Source: CAD feature listing. Evaluate the final solid. Frame: model axes, mm. A direction names the side the tool comes from. Coordinates: 2 decimals unless noted, no trailing zeros. Order: outer loops, then holes, each group sorted by start corner. A loop starts at its lowest first (then second) coordinate and runs counter-clockwise, first axis right, second up.
```python
from build123d import *

# Parameters (mm, degrees)
F1_DEPTH = 25.4
F3_DEPTH = 12.701
F5_DEPTH = 12.701


with BuildPart() as f1:
    # F0 (on Front) → F1 (new body)
    with BuildSketch(Plane.XZ):
        Polygon((-34.6547834919, 44.45), (-34.6547834919, 0), (22.4952165081, 0), (22.4952165081, 12.7), (-21.9547834919, 12.7), (-21.9547834919, 44.45), align=None)
    extrude(amount=F1_DEPTH)

    # F2 (on face) → F3 (cut, through all)
    with BuildSketch(Plane.XY.offset(12.7)):
        with BuildLine():
            ThreePointArc((-2.9047834919, -12.7), (-4.7646554313, -8.2098719395), (-9.2547834919, -6.35))
            Line((-9.2547834919, -6.35), (-9.2547834919, -19.05))
            ThreePointArc((-9.2547834919, -19.05), (-4.7646554313, -17.1901280605), (-2.9047834919, -12.7))
        make_face()
        with BuildLine():
            Line((-9.2547834919, -19.05), (-9.2547834919, -6.35))
            ThreePointArc((-9.2547834919, -6.35), (-15.6047834919, -12.7), (-9.2547834919, -19.05))
        make_face()
        with BuildLine():
            Line((9.7952165081, -19.05), (9.7952165081, -6.35))
            ThreePointArc((9.7952165081, -6.35), (3.4452165081, -12.7), (9.7952165081, -19.05))
        make_face()
        with BuildLine():
            ThreePointArc((16.1452165081, -12.7), (14.2853445687, -8.2098719395), (9.7952165081, -6.35))
            Line((9.7952165081, -6.35), (9.7952165081, -19.05))
            ThreePointArc((9.7952165081, -19.05), (14.2853445687, -17.1901280605), (16.1452165081, -12.7))
        make_face()
        with BuildLine():
            Line((22.4952165081, 0), (9.7952165081, 0))
            ThreePointArc((9.7952165081, 0), (18.7754726014, -3.7197438511), (22.4952165081, -12.6999999213))
            Line((22.4952165081, -12.6999999213), (22.4952165081, 0))
        make_face()
        with BuildLine():
            Line((22.4952165081, -25.4), (22.4952165081, -12.6999999213))
            ThreePointArc((22.4952165081, -12.6999999213), (18.775472657, -21.6802560932), (9.7952165081, -25.4))
            Line((9.7952165081, -25.4), (22.4952165081, -25.4))
        make_face()
    extrude(amount=-F3_DEPTH, mode=Mode.SUBTRACT)

    # F4 (on face) → F5 (cut, through all)
    with BuildSketch(Plane.YZ.offset(-21.9547834919)):
        with BuildLine():
            Line((-19.05, 42.7485226281), (-19.05, 31.75))
            ThreePointArc((-19.05, 31.75), (-12.7, 38.1), (-6.35, 31.75))
            Line((-6.35, 31.75), (-6.35, 42.7485226281))
            ThreePointArc((-6.35, 42.7485226281), (-9.4129981272, 44.0172579939), (-12.7, 44.45))
            ThreePointArc((-12.7, 44.45), (-15.9870018728, 44.0172579939), (-19.05, 42.7485226281))
        make_face()
        with BuildLine():
            Line((-25.4, 44.45), (-25.4, 31.75))
            ThreePointArc((-25.4, 31.75), (-23.6985226281, 38.1), (-19.05, 42.7485226281))
            ThreePointArc((-19.05, 42.7485226281), (-15.9870018728, 44.0172579939), (-12.7, 44.45))
            Line((-12.7, 44.45), (-25.4, 44.45))
        make_face()
        with BuildLine():
            Line((0, 44.45), (-12.7, 44.45))
            ThreePointArc((-12.7, 44.45), (-9.4129981272, 44.0172579939), (-6.35, 42.7485226281))
            ThreePointArc((-6.35, 42.7485226281), (-1.7014773719, 38.1), (0, 31.75))
            Line((0, 31.75), (0, 44.45))
        make_face()
        with BuildLine():
            ThreePointArc((-6.35, 31.75), (-12.7, 38.1), (-19.05, 31.75))
            Line((-19.05, 31.75), (-6.35, 31.75))
        make_face()
        with BuildLine():
            Line((-6.35, 31.75), (-19.05, 31.75))
            ThreePointArc((-19.05, 31.75), (-12.7, 25.4), (-6.35, 31.75))
        make_face()
    extrude(amount=-F5_DEPTH, mode=Mode.SUBTRACT)


solid = f1.part
```
1. Draft query along Y for faces 3 (the cylindrical face through (-28.22, -1.75, 38.18)), 4 (the flat face through (-28, -19.05, 37)), 5 (the flat face through (-18, -25.4, 9)), 6 (the flat face through (-28, -6.35, 37)). Return one class per face: +Y half, -Y half, draft (parallel to the pull), parting line (faces both ways), or undercut.
2. Section query C-C, the plane x = 8. Output: boundary loops of the cut face in (y, z), plus the area to 3 significant figures.
3. Section query B-B, the plane y = -15.5. Output: boundary loops of the cut face in (x, z).
4. Section query A-A, the plane z = 35.5. Output: boundary loops of the cut face in (x, y).
5. Access query for faces 1 (the flat face through (-18, 0, 9)), 2 (the flat face through (1, -13, 12.7)). Directions: +Z, -Z, +X, -X, +Y, -Y. A direction counts if a zero-diameter tool reaches every point of the face in a straight line with its end or side. Return the directions, or none.
6. Section query D-D, the plane z = 3. Output: boundary loops of the cut face in (x, y).
7. Material intervals for line 1 along X through (y, z) = (-13, 15.5); line 2 along Z through (x, y) = (-10, -5.75); line 3 along X through (y, z) = (-7, 11), sorted ascending.
8. Contact query for flat-ended pins moving along their axis: P1, Ø3, axis at y = -18.5, z = 19, coming from the +X side; P2, Ø10, axis at y = -21, z = 12.5, coming from the +X side; P3, Ø1, axis at x = -12.5, y = -21, coming from the +Z side. Output: stop coordinate, or through.
Answer key:
1. face 3: +Y half
1. face 4: undercut
1. face 5: -Y half
1. face 6: undercut
2. outline: (-25.4, 0) - (-18.79, 0) - (-18.79, 12.7) - (-25.4, 12.7) - close; (-6.61, 0) - (0, 0) - (0, 12.7) - (-6.61, 12.7) - close
2. area: 168 mm2
3. outline: (-34.65, 0) - (-14.95, 0) - (-14.95, 12.7) - (-21.95, 12.7) - (-21.95, 26.05) - (-34.65, 26.05) - close; (-3.56, 0) - (4.1, 0) - (4.1, 12.7) - (-3.56, 12.7) - close; (15.49, 0) - (22.18, 0) - (22.18, 12.7) - (15.49, 12.7) - close
4. outline: (-34.65, -24.83) - (-21.95, -24.83) - (-21.95, -19.05) - (-34.65, -19.05) - close; (-34.65, -6.35) - (-21.95, -6.35) - (-21.95, -0.57) - (-34.65, -0.57) - close
5. face 1: +Z, -Z, +X, -X, +Y
5. face 2: +Z, +X, +Y, -Y
6. outline: (-34.65, -25.4) - (9.8, -25.4) arc R12.7 ccw to (9.8, 0) - (-34.65, 0) - close; hole circle Ø12.7 at (-9.25, -12.7); hole circle Ø12.7 at (9.8, -12.7)
7. line 1: x = -34.65 to -21.95
7. line 2: z = 0 to 12.7
7. line 3: x = -34.65 to -12.05, -6.46 to 7, 12.59 to 21.14
8. P1: stops at x = -21.95
8. P2: stops at x = 22.06
8. P3: stops at z = 12.7
